The listing builds one solid part. Answer for the finished solid, in the listing's coordinates (mm). Coordinates: 2 decimals unless noted, no trailing zeros. Loops run counter-clockwise (first coordinate to the right, second up) from the corner with the lowest first, then second, coordinate; pieces in that order, holes last. Notation, with made-up numbers: (50, -27.75) - (104, -27.75) arc R20 cw to (104, -16.75) - close; hole circle Ø8 at (-28, 10). An arc over 180 degrees is marked (long way). Return JSON: item names as keys, results as strings. Group by question number.
1. Find the intervals of material crossed by line 1 along Y through (x, z) = (75, 0.35); line 2 along Y through (x, z) = (70, 1.1); line 3 along X through (y, z) = (55.5, 1.4), in increasing order.
2. Section A-A (z = 0.6) is taken. Write down the section's boundary in (x, y), and give its area (3 significant figures).
3. Section B-B (y = 50) is taken. Write down the section's boundary in (x, z).
4. The mould has two halves that part along X. Classify faces 1 (the face through (48, 51, 0)), 2 (the face through (65.3, 49.9, 0.8)): pulls with the +X half, pulls with the -X half, needs draft (parallel to the pull), parting line crosses it, or undercut.
```python
from build123d import *

# Parameters (mm, degrees)
SKETCH_1_W      = 98
SKETCH_1_H      = 100
EXTRUDE_1_DEPTH = 1.6
FILLET_1_R      = 2


with BuildPart() as part:
    # 草图1 → 凸台-拉伸1 (new body)
    with BuildSketch(Plane.XY):
        with Locations((49, 50)):
            Rectangle(SKETCH_1_W, SKETCH_1_H)
        with BuildLine():
            Line((96, 55), (96, 50))
            Line((96, 50), (96, 45))
            Line((96, 45), (88.8, 45))
            Line((88.8, 45), (88.8, 44))
            Line((88.8, 44), (71.3, 44))
            ThreePointArc((71.3, 44), (65.3, 50), (71.3, 56))
            Line((71.3, 56), (88.8, 56))
            Line((88.8, 56), (88.8, 55))
            Line((88.8, 55), (96, 55))
        make_face(mode=Mode.SUBTRACT)
    extrude(amount=EXTRUDE_1_DEPTH)

    # 圆角1
    fillet_1_edges = [part.edges().sort_by_distance(p)[0] for p in [
        (0, 0, 0.8),
        (0, 100, 0.8),
        (98, 100, 0.8),
        (98, 0, 0.8),
    ]]
    fillet(fillet_1_edges, radius=FILLET_1_R)


solid = part.part
```
The answers:
{
 "1": {"line 1": "y = 0 to 44, 56 to 100", "line 2": "y = 0 to 44.14, 55.86 to 100", "line 3": "x = 0 to 68.9, 88.8 to 98"},
 "2": {"outline": "(0, 2) arc R2 ccw to (2, 0) - (96, 0) arc R2 ccw to (98, 2) - (98, 98) arc R2 ccw to (96, 100) - (2, 100) arc R2 ccw to (0, 98) - close; hole (71.3, 44) - (88.8, 44) - (88.8, 45) - (96, 45) - (96, 55) - (88.8, 55) - (88.8, 56) - (71.3, 56) arc R6 ccw to start", "area": "9,460 mm2"},
 "3": {"outline": "(0, 0) - (65.3, 0) - (65.3, 1.6) - (0, 1.6) - close; (96, 0) - (98, 0) - (98, 1.6) - (96, 1.6) - close"},
 "4": {"face 1": "needs draft", "face 2": "undercut"}
}
